```python
from build123d import *

# Parameters (mm, degrees)
CROQUIS1_R              = 15
CROQUIS1_R_2            = 9
SALIENTE_EXTRUIR1_DEPTH = 25
CROQUIS2_R              = 10.95
CORTAR_EXTRUIR1_DEPTH   = 7
CROQUIS3_R              = 1.6
SALIENTE_EXTRUIR2_DEPTH = 4
CORTAR_EXTRUIR2_DEPTH   = 26
MATRIZC1_COUNT          = 4


with BuildPart() as part:
    # Croquis1 → Saliente-Extruir1 (new body)
    with BuildSketch(Plane(origin=(0, 0, 0), x_dir=(0, 1, 0), z_dir=(0, 0, 1))):
        with Locations(Location((0, 0, 0), (0, 0, 270))):
            Circle(CROQUIS1_R)
        with Locations(Location((0, 0, 0), (0, 0, 270))):
            Circle(CROQUIS1_R_2, mode=Mode.SUBTRACT)
    extrude(amount=SALIENTE_EXTRUIR1_DEPTH)

    # Croquis2 → Cortar-Extruir1 (cut)
    with BuildSketch(Plane.XY.offset(25)):
        Circle(CROQUIS2_R)
    extrude(amount=-CORTAR_EXTRUIR1_DEPTH, mode=Mode.SUBTRACT)

    # Croquis3 → Saliente-Extruir2 (add)
    with BuildSketch(Plane(origin=(0, 0, 0), x_dir=(0, 1, 0), z_dir=(0, 0, 1))):
        with BuildLine():
            Line((-20.000196267, -2.236419092), (-9.999672874, -11.180632469))
            ThreePointArc((-9.999672874, -11.180632469), (-15, 0), (-9.999672874, 11.180632469))
            Line((-9.999672874, 11.180632469), (-20.000196267, 2.236419092))
            ThreePointArc((-20.000196267, 2.236419092), (-21.000392551, 0), (-20.000196267, -2.236419092))
        make_face()
        with Locations(Location((-18, 0, 0), (0, 0, 270))):
            Circle(CROQUIS3_R, mode=Mode.SUBTRACT)
    saliente_extruir2 = extrude(amount=SALIENTE_EXTRUIR2_DEPTH)

    # Simetría1: Saliente-Extruir2 across plane
    add(saliente_extruir2.mirror(Plane.ZX))

    # Croquis4 → Cortar-Extruir2 (cut)
    with BuildSketch(Plane.YZ):
        with BuildLine():
            Line((-2, 8), (-2, 13))
            ThreePointArc((-2, 13), (0, 15), (2, 13))
            Line((2, 13), (2, 8))
            ThreePointArc((2, 8), (0, 6), (-2, 8))
        make_face()
    cortar_extruir2 = extrude(amount=-CORTAR_EXTRUIR2_DEPTH, mode=Mode.SUBTRACT)

    # MatrizC1: Cortar-Extruir2 ×4 about axis
    matrizc1_axis = Axis((0, 0, 0), (0, 0, 1))
    for i in range(1, MATRIZC1_COUNT):
        add(cortar_extruir2.rotate(matrizc1_axis, i * 360 / MATRIZC1_COUNT), mode=Mode.SUBTRACT)


solid = part.part
```
Verification items for the finished model (mm, model axes). A direction names the side the tool comes from. Give positions to 0.01 mm unless a question says otherwise; leave off trailing zeros. Order: outer loops, then holes, each group sorted by start corner. A loop starts at its lowest first (then second) coordinate and runs counter-clockwise, first axis right, second up. Notation, with made-up numbers: M 73.25,66.25 L 84.25,66.25 A13 cw 84.25,83.25 Z; hole C 9,42 d4. An arc over 180 degrees is marked long. Return JSON: item names as keys, results as strings. Group by question number.
1) Section check B-B on x = 0. Give the number of separate pieces and of enclosed holes in the cut face, and give its area (3 significant figures).
2) Section check D-D on y = 8. Record the cut outline in (x, z), and give its area (3 significant figures).
3) Section check C-C on z = 10.5. Record the cut outline in (x, y), and give its area (3 significant figures).
4) Access from +Z, -Z, +X, -X, +Y, -Y to the whole of each face (thin tool, end or side, straight path). Record for faces 1 (the face through (3, -9, 0)), 2 (the face through (0, 12, 6)), 3 (the face through (12, -2, 11)).
5) Mould release check, pull along Y, two halves, no side actions. Record for faces 4 (the face through (6.646, -15.07, 1.972)), 5 (the face through (1, -16, 4)), 6 (the face through (-2, -9, 18)), 7 (the face through (8.314, -3.447, 8.874)): pulls with the +Y half, pulls with the -Y half, needs draft (parallel to the pull), parting line crosses it, or undercut.
6) Go/stop test with flat-tipped pins: pin 1 Ø2.5 at (x, y) = (0, 18) entering from +Z; pin 2 Ø3 at (x, z) = (2.5, 10) entering from +Y; pin 3 Ø5.5 at (x, z) = (-11, 9.5) entering from -Y; pin 4 Ø6 at (x, z) = (7.5, 14) entering from -Y. Record where each tip stops, or that it passes through.
7) Section check A-A on y = 0. Record the cut outline in (x, z).
8) Scan lines: line 1 (Y direction, x = 0, z = 2.65); line 2 (Y direction, x = 0, z = 19.25); line 3 (X direction, y = 0, z = 4). Record each from-to range of solid material in increasing order.
Answer block:
{
 "1": {"separate pieces": "6", "enclosed holes": "0", "area": "187 mm^2"},
 "2": {"outline": "M -12.69,0 L -4.12,0 L -4.12,18 L -7.48,18 L -7.48,25 L -12.69,25 Z; M 4.12,0 L 12.69,0 L 12.69,25 L 7.48,25 L 7.48,18 L 4.12,18 Z", "area": "381 mm^2"},
 "3": {"outline": "M -14.87,-2 A15 ccw -2,-14.87 L -2,-8.77 A9 cw -8.77,-2 Z; M -14.87,2 L -8.77,2 A9 cw -2,8.77 L -2,14.87 A15 ccw Z; M 2,-14.87 A15 ccw 14.87,-2 L 8.77,-2 A9 cw 2,-8.77 Z; M 2,8.77 A9 cw 8.77,2 L 14.87,2 A15 ccw 2,14.87 Z", "area": "356 mm^2"},
 "4": {"face 1": "-Z, +X, -X, +Y, -Y", "face 2": "+Y, -Y", "face 3": "+X, -X"},
 "5": {"face 4": "pulls with the -Y half", "face 5": "needs draft", "face 6": "undercut", "face 7": "undercut"},
 "6": {"pin 1": "passes through", "pin 2": "stops at y = 14.87", "pin 3": "stops at y = -12.53", "pin 4": "stops at y = -14.31"},
 "7": {"outline": "M -15,0 L -9,0 L -9,6 L -15,6 Z; M -15,15 L -9,15 L -9,18 L -10.95,18 L -10.95,25 L -15,25 Z; M 9,0 L 15,0 L 15,6 L 9,6 Z; M 9,15 L 15,15 L 15,25 L 10.95,25 L 10.95,18 L 9,18 Z"},
 "8": {"line 1": "y = -21 to -19.6, -16.4 to -9, 9 to 16.4, 19.6 to 21", "line 2": "y = -15 to -10.95, 10.95 to 15", "line 3": "x = -15 to -9, 9 to 15"}
}
